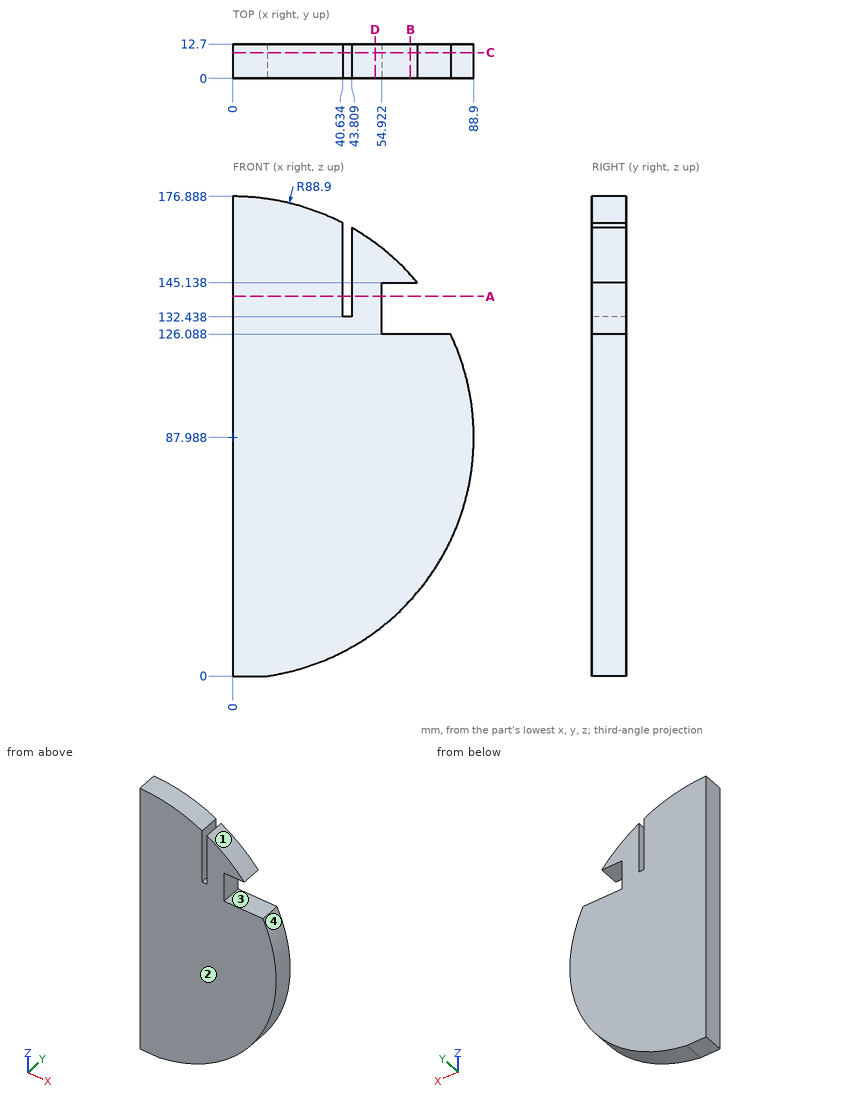
The figure shows three views and two pictorial views of one solid part (mm, origin at its lowest corner). Answer the questions. Round coordinates to 2 decimals unless told otherwise and drop trailing zeros. Write each loop counter-clockwise with the first axis right and the second up, starting at its lowest first coordinate (ties: lowest second). Pieces come first, ordered by that corner, then holes. Notation, with made-up numbers: (24.25, 30) -> (40.25, 30) arc R9 ccw to (40.25, 45) -> close; hole circle Ø2 at (48.5, 2). An arc over 180 degrees is marked (long way). Answer as a JSON object with one key per item and string values. Group by question number.
Q1. Section C-C (y = 9.5) is taken. Write down the section's boundary in (x, z) (1 decimal), plus the area to 3 significant figures.
Q2. Section B-B (x = 65.5) is taken. Write down the section's boundary in (y, z).
Q3. Section A-A (z = 140) is taken. Write down the section's boundary in (x, y) (1 decimal).
Q4. Each of these flat-tipped pins is pushed along its axis until it touches: pin 1 Ø3.5 at (x, y) = (42, 4.5) entering from +Z (1 decimal); pin 2 Ø6 at (x, y) = (32, 4.5) entering from -Z; pin 3 Ø4 at (x, y) = (63.5, 8) entering from -Z. Where does it stop, or does it pass through?
Q5. Determine the mould class of the marked faces 1, 2, 3 and 4 for opening direction Z: pulls with the +Z half, pulls with the -Z half, needs draft (parallel to the pull), parting line crosses it, or undercut.
Q6. Section D-D (x = 52.5) is taken. Write down the section's boundary in (y, z), plus the area to 3 significant figures.
Q7. Straight lines are drawn through the part: line 1 along X through (y, z) = (7.25, 140.5) (1 decimal); line 2 along X through (y, z) = (4.75, 153.5) (1 decimal); line 3 along X through (y, z) = (8, 128). For each, find the intervals that lie inside material, in ascending order.
Check values:
{
 "1": {"outline": "(0, 0) -> (12.7, 0) arc R88.9 ccw to (80.3, 126.1) -> (54.9, 126.1) -> (54.9, 145.1) -> (68.1, 145.1) arc R88.9 ccw to (43.8, 165.3) -> (43.8, 132.4) -> (40.6, 132.4) -> (40.6, 167.1) arc R88.9 ccw to (0, 176.9) -> close", "area": "11,900 mm^2"},
 "2": {"outline": "(0, 27.88) -> (12.7, 27.88) -> (12.7, 126.09) -> (0, 126.09) -> close; (0, 145.14) -> (12.7, 145.14) -> (12.7, 148.1) -> (0, 148.1) -> close"},
 "3": {"outline": "(0, 0) -> (40.6, 0) -> (40.6, 12.7) -> (0, 12.7) -> close; (43.8, 0) -> (54.9, 0) -> (54.9, 12.7) -> (43.8, 12.7) -> close"},
 "4": {"pin 1": "z = 167.3", "pin 2": "z = 3.95", "pin 3": "z = 23.79"},
 "5": {"face 1": "pulls with the +Z half", "face 2": "needs draft", "face 3": "undercut", "face 4": "parting line crosses it"},
 "6": {"outline": "(0, 16.25) -> (12.7, 16.25) -> (12.7, 159.73) -> (0, 159.73) -> close", "area": "1,820 mm^2"},
 "7": {"line 1": "0 to 40.6, 43.8 to 54.9", "line 2": "0 to 40.6, 43.8 to 60.1", "line 3": "0 to 54.92"}
}
